Work out the finished part from the listing and answer in its coordinate system (mm). A direction names the side the tool comes from. Round coordinates to 2 decimals unless told otherwise and drop trailing zeros. Loops run counter-clockwise (first coordinate to the right, second up) from the corner with the lowest first, then second, coordinate; pieces in that order, holes last. Notation, with made-up numbers: (40.25, -19.5) - (92.25, -19.5) arc R28 cw to (92.25, 2.5) - close; hole circle Ø4 at (-37.75, 53.5). An arc over 180 degrees is marked (long way). Answer as CSV lines item,"result". Start each with the question number.
Q1. Section B-B on x = 0 is taken. Write down the section's boundary in (y, z), then the cut area to 3 significant figures.
Q2. For faces 5 (the face through (-2, 65, 22)), 6 (the face through (9, 36, 18)), determine the directions among +Z, -Z, +X, -X, +Y, -Y from which every point of the face is accessible in a straight line to the end or side of a thin tool.
Q3. The mould has two halves that part along Y. Classify faces 1 (the face through (-122.5, -2, 11)), 2 (the face through (-8.201, 51.364, 20.028)), 3 (the face through (-1.7, -135.9, 11.2)), 4 (the face through (-2, 138.9, 11)): +Y half, -Y half, draft (parallel to the pull), parting line (faces both ways), or undercut.
Q4. Straight lines are drawn through the part: L1, parallel to Y at x = -43, z = 13.5; L2, parallel to Y at x = 0, z = 19.05; L3, parallel to X at y = -38.5, z = 1.75. For each, find the intervals that lie inside material, in ascending order. Write a range as [from, to].
Q5. Each of these flat-tipped pins is pushed along its axis until it touches: pin 1 Ø6 at (x, y) = (-48.5, -15.5) entering from +Z; pin 2 Ø3 at (x, z) = (29, 13) entering from -Y; pin 3 Ø4 at (x, z) = (60, 7.5) entering from -Y. Where does it stop, or does it pass through?
Q6. Section A-A on y = -11.1 is taken. Write down the section's boundary in (x, z).
Q7. Section C-C on z = 6.5 is taken. Write down the section's boundary in (x, y), then the cut area to 3 significant figures.
```python
from build123d import *

# Parameters (mm, degrees)
F0_W     = 245
F0_H     = 277.8
F1_DEPTH = 22
F3_D     = 95
F4_R     = 63
F5_DEPTH = 4
F7_DEPTH = 245.001


with BuildPart() as f1:
    # F0 (on Top) → F1 (new body)
    with BuildSketch(Plane.XY):
        Rectangle(F0_W, F0_H)
    extrude(amount=F1_DEPTH)

    # F3 (through all)
    with Locations(Plane.XY.offset(22)):
        with Locations((0, -11.1)):
            Hole(F3_D / 2)

    # F4 (on face) → F5 (cut)
    with BuildSketch(Plane.XY.offset(22)):
        with Locations((0, -11.1)):
            Circle(F4_R)
    extrude(amount=-F5_DEPTH, mode=Mode.SUBTRACT)

    # F6 (on face) → F7 (cut, through all)
    with BuildSketch(Plane(origin=(-122.5, 0, 0), x_dir=(0, -1, 0), z_dir=(-1, 0, 0))):
        Polygon((133.005118, 22), (138.9, 0), (138.9, 22), align=None)
    extrude(amount=-F7_DEPTH, mode=Mode.SUBTRACT)


solid = f1.part
```
Findings:
1,outline,"(-138.9, 0) - (-58.6, 0) - (-58.6, 18) - (-74.1, 18) - (-74.1, 22) - (-133.01, 22) - close; (36.4, 0) - (138.9, 0) - (138.9, 22) - (51.9, 22) - (51.9, 18) - (36.4, 18) - close"
1,area,"3,830 mm^2"
2,face 5,"+Z, +X, -X, +Y, -Y"
2,face 6,"+Z"
3,face 1,"draft"
3,face 2,"undercut"
3,face 3,"-Y half"
3,face 4,"+Y half"
4,L1,"y = [-135.28, -31.28], [9.08, 138.9]"
4,L2,"y = [-133.8, -74.1], [51.9, 138.9]"
4,L3,"x = [-122.5, -38.8], [38.8, 122.5]"
5,pin 1,"stops at z = 18"
5,pin 2,"stops at y = -135.82"
5,pin 3,"stops at y = -137.43"
6,outline,"(-122.5, 0) - (-47.5, 0) - (-47.5, 18) - (-63, 18) - (-63, 22) - (-122.5, 22) - close; (47.5, 0) - (122.5, 0) - (122.5, 22) - (63, 22) - (63, 18) - (47.5, 18) - close"
7,outline,"(-122.5, -137.16) - (122.5, -137.16) - (122.5, 138.9) - (-122.5, 138.9) - close; hole circle Ø95 at (0, -11.1)"
7,area,"60,500 mm^2"
